Geometry: final body of the model. Coordinates: model frame, mm. A direction names the side the tool comes from. Round coordinates to 2 decimals unless told otherwise and drop trailing zeros. Write each loop counter-clockwise with the first axis right and the second up, starting at its lowest first coordinate (ties: lowest second). Pieces come first, ordered by that corner, then holes. Notation, with made-up numbers: M 67,33 L 91,33 A15 ccw 91,53 Z; hole C 21.25,62 d8. An arc over 180 degrees is marked long. Use one line per item in the form item = value. Start each with the question number.
Item 1: Section query C-C (z = -0.5). State how many separate pieces and enclosed holes the cut face has, and give its area (3 significant figures).
Item 2: Section query A-A (x = 15). Return loops of the section in (y, z), and give its area (3 significant figures).
Item 3: Reachability of faces 1 (the cylindrical face through (-66, 11, 0)), 2 (the flat face through (-58, 14.5, -7)), 3 (the cylindrical face through (-22.479, 15.476, 4.967)), 4 (the flat face through (-55, 5.5, 0)) from +Z, -Z, +X, -X, +Y, -Y: full face, straight path, thin tool, end or side. Return the list, or none.
Item 4: Section query D-D (x = -1). Return loops of the section in (y, z), and give its area (3 significant figures).
Item 5: Pull-direction query (Y, two-part tool) for faces 5 (the flat face through (-58, 14.5, 7)), 6 (the cylindrical face through (1.82, 7.96, 1.45)), 7 (the flat face through (24, 7, 0)); classes: pulls with the +Y half, pulls with the -Y half, needs draft (parallel to the pull), parting line crosses it, or undercut.
Item 6: Ray query, probe 1 along Y at (x, z) = (-8, 0); probe 2 along Y at (x, z) = (-22.6, -4.75); probe 3 along Y at (x, z) = (14.5, 0.5). Return the intervals inside material, ascending.
Item 7: Section query B-B (y = 16.5). Return loops of the section in (x, z).
Item 8: Pin query (flat end, axial travel): pin 1 Ø3 at (y, z) = (20, 3) entering from -X; pin 2 Ø1.9 at (x, z) = (-60, -6.5) entering from -Y; pin 3 Ø10 at (y, z) = (16, 6.5) entering from -X; pin 4 Ø6 at (x, z) = (-41, 5) entering from -Y. Return the tip coordinate at first contact, or that it passes through.
from build123d import *

# Parameters (mm, degrees)
SKETCH_1_W          = 48
SKETCH_1_H          = 18
EXTRUDE_1_DEPTH     = 3.5
SKETCH_6_W          = 18
SKETCH_6_H          = 9
EXTRUDE_4_DEPTH     = 23
SKETCH_7_R          = 3.5
CUT_EXTRUDE_1_DEPTH = 2
SKETCH_9_R          = 5.5
CUT_EXTRUDE_4_DEPTH = 3
CUT_EXTRUDE_5_REACH = 75.995
SKETCH_10_R         = 7.5
CUT_EXTRUDE_6_REACH = 71.957
SKETCH_11_R         = 1.6
EXTRUDE_5_OUTLINE_W = 48
EXTRUDE_5_OUTLINE_H = 18
EXTRUDE_5_DEPTH     = 20
CUT_EXTRUDE_7_REACH = 96.415
SKETCH_13_R         = 3.25
SKETCH_13_R_2       = 1
SKETCH_15_R         = 6.7
CUT_EXTRUDE_8_DEPTH = 45
SKETCH_16_R         = 3.15
CUT_EXTRUDE_9_DEPTH = 74.247867011


with BuildPart() as part:
    # 草圖1 → 填料-伸長1 (new, symmetric)
    with BuildSketch(Plane(origin=(0, 0, 0), x_dir=(1, 0, 0), z_dir=(0, 1, 0))):
        Rectangle(SKETCH_1_W, SKETCH_1_H)
    extrude(amount=EXTRUDE_1_DEPTH, both=True)

    # Sketch 3D_3 → Loft 1 section 0
    with BuildSketch(Plane(origin=(-44, 14.5, -9), x_dir=(0, -0.447213595499958, 0.894427190999916), z_dir=(-1, 0, 0))):
        with BuildLine():
            Line((0, 0), (16.099689438, 8.049844719))
            Line((16.099689438, 8.049844719), (20.124611797, 0))
            Line((20.124611797, 0), (4.024922359, -8.049844719))
            Line((4.024922359, -8.049844719), (0, 0))
        make_face()
    # 草圖5 → Loft 1 section 1
    with BuildSketch(Plane.ZY.offset(24)):
        with BuildLine():
            Line((-9, 3.5), (9, 3.5))
            Line((9, 3.5), (9, -3.5))
            Line((9, -3.5), (-9, -3.5))
            Line((-9, -3.5), (-9, 3.5))
        make_face()
    loft()

    # 草圖6 → 填料-伸長4 (add)
    with BuildSketch(Plane.ZY.offset(44)):
        with Locations((0, 10)):
            Rectangle(SKETCH_6_W, SKETCH_6_H)
    extrude(amount=EXTRUDE_4_DEPTH)

    # 草圖7 → 除料-伸長1 (cut)
    with BuildSketch(Plane.ZY.offset(67)):
        with Locations((0, 14.5)):
            Circle(SKETCH_7_R)
    extrude(amount=-CUT_EXTRUDE_1_DEPTH, mode=Mode.SUBTRACT)

    # Loft 1 2: read off the stored shape, not the designer's step
    # Loft 1 2: loft between two sections, ruled curve by curve
    loft_1_2_from = [
        Edge.make_bspline([(-65, 14.5, 3.5), (-65, 12.75, 3.5), (-65, 11, 2.333333333), (-65, 11, -2.333333333), (-65, 12.75, -3.5), (-65, 14.5, -3.5)], [0, 0, 0, 0, 0.5, 0.5, 1, 1, 1, 1], 3, [1, 0.666666667, 0.5, 0.5, 0.666666667, 1]),
        Edge.make_line((-65, 14.5, -3.5), (-65, 14.5, 3.5)),
    ]
    loft_1_2_to = [
        Edge.make_bspline([(-53, 15.833945938, 5.335783751), (-53, 12.063417219, 6.27841593), (-53, 9, 3.886572043), (-53, 9, -3.886572043), (-53, 12.063417219, -6.27841593), (-53, 15.833945938, -5.335783751)], [0, 0, 0, 0, 0.5, 0.5, 1, 1, 1, 1], 3, [1, 0.552953065, 0.4111804, 0.4111804, 0.552953065, 1]),
        Edge.make_line((-53, 15.833945938, -5.335783751), (-53, 15.833945938, 5.335783751)),
    ]
    loft_1_2 = Solid(Shell([*[Face.make_surface_from_curves(loft_1_2_from[k], loft_1_2_to[k]) for k in range(2)], Face(Wire(loft_1_2_from)), Face(Wire(loft_1_2_to))]))
    add(loft_1_2, mode=Mode.SUBTRACT)

    # 草圖9 → 除料-伸長4 (cut)
    with BuildSketch(Plane.ZY.offset(53)):
        with Locations((3.554e-06, 14.500000002)):
            Circle(SKETCH_9_R)
    extrude(amount=-CUT_EXTRUDE_4_DEPTH, mode=Mode.SUBTRACT)

    # 除料-疊層拉伸4: read off the stored shape, not the designer's step
    # 除料-疊層拉伸4: loft between two sections, ruled curve by curve
    loft_4_from = [
        Edge.make_bspline([(-50, 14.5, 5.500003554), (-50, 11.750000001, 5.500003553), (-50, 9.000000002, 3.66667022), (-50, 9.000000002, -3.666663111), (-50, 11.750000001, -5.499996445), (-50, 14.5, -5.499996446)], [0, 0, 0, 0, 0.5, 0.5, 1, 1, 1, 1], 3, [1, 0.666666667, 0.5, 0.5, 0.666666667, 1]),
        Edge.make_line((-50, 14.5, -5.499996446), (-50, 14.5, 5.500003554)),
    ]
    loft_4_to = [
        Edge.make_bspline([(-48, 16.319017189, 7.276072306), (-48, 11.177387119, 8.561479823), (-48, 7.000000002, 5.299874521), (-48, 7.000000002, -5.299867413), (-48, 11.177387119, -8.561472714), (-48, 16.319017189, -7.276065197)], [0, 0, 0, 0, 0.5, 0.5, 1, 1, 1, 1], 3, [1, 0.552953065, 0.4111804, 0.4111804, 0.552953065, 1]),
        Edge.make_line((-48, 16.319017189, -7.276065197), (-48, 16.319017189, 7.276072306)),
    ]
    loft_4 = Solid(Shell([*[Face.make_surface_from_curves(loft_4_from[k], loft_4_to[k]) for k in range(2)], Face(Wire(loft_4_from)), Face(Wire(loft_4_to))]))
    add(loft_4, mode=Mode.SUBTRACT)

    # 草圖10 → 除料-伸長5 (cut, up to next)
    with BuildSketch(Plane.ZY.offset(48), mode=Mode.PRIVATE) as cut_extrude_5_sk1:
        with Locations((4.786e-06, 14.500000002)):
            Circle(SKETCH_10_R)
    cut_extrude_5_tool1 = extrude(cut_extrude_5_sk1.sketch, amount=-CUT_EXTRUDE_5_REACH, mode=Mode.PRIVATE) & part.part
    add(cut_extrude_5_tool1.solids().sort_by_distance((-48, 14.5, 5e-06))[0], mode=Mode.SUBTRACT)

    # 草圖11 → 除料-伸長6 (cut, up to next)
    with BuildSketch(Plane(origin=(0, 14.5, 0), x_dir=(1, 0, 0), z_dir=(0, 1, 0)), mode=Mode.PRIVATE) as cut_extrude_6_sk1:
        with Locations(Location((-60, -6.5, 0), (0, 0, 270))):
            Circle(SKETCH_11_R)
    cut_extrude_6_tool1 = extrude(cut_extrude_6_sk1.sketch, amount=-CUT_EXTRUDE_6_REACH, mode=Mode.PRIVATE) & part.part
    # 草圖11 → 除料-伸長6 (cut, up to next)
    with BuildSketch(Plane(origin=(0, 14.5, 0), x_dir=(1, 0, 0), z_dir=(0, 1, 0)), mode=Mode.PRIVATE) as cut_extrude_6_sk2:
        with Locations(Location((-60, 6.5, 0), (0, 0, 270))):
            Circle(SKETCH_11_R)
    cut_extrude_6_tool2 = extrude(cut_extrude_6_sk2.sketch, amount=-CUT_EXTRUDE_6_REACH, mode=Mode.PRIVATE) & part.part
    add(cut_extrude_6_tool1.solids().sort_by_distance((-60, 14.5, 6.5))[0], mode=Mode.SUBTRACT)
    add(cut_extrude_6_tool2.solids().sort_by_distance((-60, 14.5, -6.5))[0], mode=Mode.SUBTRACT)

    # 填料-伸長5: read off the stored shape, not the designer's step
    # 填料-伸長5 outline → 填料-伸長5 (add)
    with BuildSketch(Plane(origin=(0, 3.5, 0), x_dir=(1, 0, 0), z_dir=(0, 1, 0))):
        Rectangle(EXTRUDE_5_OUTLINE_W, EXTRUDE_5_OUTLINE_H)
    extrude(amount=EXTRUDE_5_DEPTH)

    # 草圖13 → 除料-伸長7 (cut, up to next)
    with BuildSketch(Plane.ZY.offset(-24), mode=Mode.PRIVATE) as cut_extrude_7_sk1:
        with Locations(Location((0, 14.5, 0), (0, 0, 180))):
            Circle(SKETCH_13_R)
    cut_extrude_7_tool1 = extrude(cut_extrude_7_sk1.sketch, amount=CUT_EXTRUDE_7_REACH, mode=Mode.PRIVATE) & part.part
    # 草圖13 → 除料-伸長7 (cut, up to next)
    with BuildSketch(Plane.ZY.offset(-24), mode=Mode.PRIVATE) as cut_extrude_7_sk2:
        with Locations(Location((-4.75, 14.5, 0), (0, 0, 180))):
            Circle(SKETCH_13_R_2)
    cut_extrude_7_tool2 = extrude(cut_extrude_7_sk2.sketch, amount=CUT_EXTRUDE_7_REACH, mode=Mode.PRIVATE) & part.part
    # 草圖13 → 除料-伸長7 (cut, up to next)
    with BuildSketch(Plane.ZY.offset(-24), mode=Mode.PRIVATE) as cut_extrude_7_sk3:
        with Locations(Location((4.75, 14.5, 0), (0, 0, 180))):
            Circle(SKETCH_13_R_2)
    cut_extrude_7_tool3 = extrude(cut_extrude_7_sk3.sketch, amount=CUT_EXTRUDE_7_REACH, mode=Mode.PRIVATE) & part.part
    add(cut_extrude_7_tool1.solids().sort_by_distance((24, 14.5, 0))[0], mode=Mode.SUBTRACT)
    add(cut_extrude_7_tool2.solids().sort_by_distance((24, 14.5, -4.75))[0], mode=Mode.SUBTRACT)
    add(cut_extrude_7_tool3.solids().sort_by_distance((24, 14.5, 4.75))[0], mode=Mode.SUBTRACT)

    # 草圖15 → 除料-伸長8 (cut)
    with BuildSketch(Plane(origin=(24, 0, 0), x_dir=(0, 0, -1), z_dir=(1, 0, 0))):
        with Locations((0, 14.5)):
            Circle(SKETCH_15_R)
    extrude(amount=-CUT_EXTRUDE_8_DEPTH, mode=Mode.SUBTRACT)

    # 草圖16 → 除料-伸長9 (cut, through all)
    with BuildSketch(Plane.XY.offset(9)):
        with Locations((15, 2.5)):
            Circle(SKETCH_16_R)
        with Locations((0, 2.5)):
            Circle(SKETCH_16_R)
        with Locations((-15, 2.5)):
            Circle(SKETCH_16_R)
    extrude(amount=-CUT_EXTRUDE_9_DEPTH, mode=Mode.SUBTRACT)


solid = part.part
Working result:
q1.separate_pieces = 2
q1.enclosed_holes = 3
q1.area = 778 mm²
q2.outline = M -3.5,-9 L -0.65,-9 L -0.65,9 L -3.5,9 Z; M 5.65,-9 L 23.5,-9 L 23.5,9 L 5.65,9 Z; hole C 14.5,0 d13.4
q2.area = 232 mm²
q3.face_1 = -X, +Y
q3.face_2 = +Z, -Z, -X, +Y
q3.face_3 = +X
q3.face_4 = +Z, -Z, -X, -Y
q4.outline = M -3.5,-9 L -0.49,-9 L -0.49,9 L -3.5,9 Z; M 5.49,-9 L 23.5,-9 L 23.5,9 L 5.49,9 Z; hole C 14.5,0 d13.4
q4.area = 237 mm²
q5.face_5 = pulls with the +Y half
q5.face_6 = undercut
q5.face_7 = needs draft
q6.probe_1 = -3.5 to 7.8, 21.2 to 23.5
q6.probe_2 = -3.5 to 13.5, 15.5 to 23.5
q6.probe_3 = -3.5 to -0.61, 5.61 to 7.82, 21.18 to 23.5
q7.outline = M -24,-9 L 24,-9 L 24,-6.39 L -21,-6.39 L -21,-2.56 L -24,-2.56 Z; M -24,2.56 L -21,2.56 L -21,6.39 L 24,6.39 L 24,9 L -24,9 Z
q8.pin_1 = -24
q8.pin_2 = through
q8.pin_3 = -67
q8.pin_4 = 2.8
